Could you check a few things on this model? Use its own coordinates, in mm. A direction names the side the tool comes from. Give positions to 0.01 mm unless a question says otherwise; leave off trailing zeros. Write each loop counter-clockwise with the first axis right and the second up, starting at its lowest first coordinate (ties: lowest second). Pieces come first, ordered by that corner, then holes. Notation, with made-up numbers: M 23,53 L 33,53 A32 ccw 33,88 Z; hole C 79.5,-13.75 d6. An arc over 180 degrees is marked long. One line per item, written item: value.
```python
from build123d import *
from OCP.BRepFilletAPI import BRepFilletAPI_MakeChamfer

# Parameters (mm, degrees)
BOSS_EXTRUDE1_DEPTH      = 7
SKETCH2_R                = 1.5
CUT_EXTRUDE1_DEPTH       = 43.613787576
SKETCH3_R                = 1.5
CUT_EXTRUDE2_DEPTH       = 5
CHAMFER1_SIZE            = 0.5
CHAMFER1_SIZE2           = 0.595876796
BOSS_EXTRUDE2_DEPTH      = 2.5
BOSS_EXTRUDE2_DEPTH_BACK = 2.5
FILLET1_R                = 5
FILLET2_START            = -2.004201681
FILLET2_DEPTH            = 7.008403362
FILLET2_START_2          = 15
FILLET2_2_DEPTH          = 3


with BuildPart() as part:
    # Sketch1 → Boss-Extrude1 (new body)
    with BuildSketch(Plane(origin=(0, 0, 0), x_dir=(1, 0, 0), z_dir=(0, 1, 0))):
        with BuildLine():
            Line((15, 2.004201681), (-15, 2.004201681))
            Line((-15, 2.004201681), (-15, -2.004201681))
            Line((-15, -2.004201681), (-4, -2.004201681))
            Line((-4, -2.004201681), (-4, -37.495798319))
            Line((-4, -37.495798319), (-1, -37.495798319))
            Line((-1, -37.495798319), (-1, -30.895798319))
            ThreePointArc((-1, -30.895798319), (0, -25.895798319), (1, -30.895798319))
            Line((1, -30.895798319), (1, -37.495798319))
            Line((1, -37.495798319), (4, -37.495798319))
            Line((4, -37.495798319), (4, -2.004201681))
            Line((4, -2.004201681), (15, -2.004201681))
            Line((15, -2.004201681), (15, 2.004201681))
        make_face()
    extrude(amount=BOSS_EXTRUDE1_DEPTH)

    # Sketch2 → Cut-Extrude1 (cut, through all)
    with BuildSketch(Plane(origin=(4, 0, 0), x_dir=(0, 0, -1), z_dir=(1, 0, 0))):
        with Locations((-33.395798319, 3.5)):
            Circle(SKETCH2_R)
    extrude(amount=-CUT_EXTRUDE1_DEPTH, mode=Mode.SUBTRACT)

    # Sketch3 → Cut-Extrude2 (cut)
    with BuildSketch(Plane.XY.offset(2.004201681)):
        with Locations((9, 3.5)):
            Circle(SKETCH3_R)
        with Locations(Location((-9, 3.5, 0), (0, 0, 180))):
            Circle(SKETCH3_R)
    extrude(amount=-CUT_EXTRUDE2_DEPTH, mode=Mode.SUBTRACT)

    # Chamfer1: one chamfer whose edges measure the first distance from different faces: ONE call of the kernel's chamfer builder (chamfer() names one face for all edges)
    chamfer1_edges_1 = [part.edges().sort_by_distance(p)[0] for p in [
        (-1, 0, 34.195798319),
    ]]
    chamfer1_side_1 = [part.faces().sort_by_distance(p)[0] for p in [
        (-1, 3.5, 37.399590212),
    ]]
    chamfer1_edges_2 = [part.edges().sort_by_distance(p)[0] for p in [
        (-2.5, 0, 37.495798319),
    ]]
    chamfer1_side_2 = [part.faces().sort_by_distance(p)[0] for p in [
        (-2.5, 3.5, 37.495798319),
    ]]
    chamfer1_edges_3 = [part.edges().sort_by_distance(p)[0] for p in [
        (-4, 0, 19.75),
    ]]
    chamfer1_side_3 = [part.faces().sort_by_distance(p)[0] for p in [
        (-4, 3.5, 19.350383526),
    ]]
    chamfer1_edges_4 = [part.edges().sort_by_distance(p)[0] for p in [
        (-9.5, 0, 2.004201681),
    ]]
    chamfer1_side_4 = [part.faces().sort_by_distance(p)[0] for p in [
        (-14.869615952, 3.5, 2.004201681),
    ]]
    chamfer1_edges_5 = [part.edges().sort_by_distance(p)[0] for p in [
        (-15, 0, 0),
    ]]
    chamfer1_side_5 = [part.faces().sort_by_distance(p)[0] for p in [
        (-15, 3.5, 0),
    ]]
    chamfer1_edges_6 = [part.edges().sort_by_distance(p)[0] for p in [
        (0, 0, -2.004201681),
    ]]
    chamfer1_side_6 = [part.faces().sort_by_distance(p)[0] for p in [
        (0, 3.5, -2.004201681),
    ]]
    chamfer1_edges_7 = [part.edges().sort_by_distance(p)[0] for p in [
        (15, 0, 0),
    ]]
    chamfer1_side_7 = [part.faces().sort_by_distance(p)[0] for p in [
        (15, 3.5, 0),
    ]]
    chamfer1_edges_8 = [part.edges().sort_by_distance(p)[0] for p in [
        (9.5, 0, 2.004201681),
    ]]
    chamfer1_side_8 = [part.faces().sort_by_distance(p)[0] for p in [
        (4.130384048, 3.5, 2.004201681),
    ]]
    chamfer1_edges_9 = [part.edges().sort_by_distance(p)[0] for p in [
        (4, 0, 19.75),
    ]]
    chamfer1_side_9 = [part.faces().sort_by_distance(p)[0] for p in [
        (4, 3.5, 19.350383526),
    ]]
    chamfer1_edges_10 = [part.edges().sort_by_distance(p)[0] for p in [
        (2.5, 0, 37.495798319),
    ]]
    chamfer1_side_10 = [part.faces().sort_by_distance(p)[0] for p in [
        (2.5, 3.5, 37.495798319),
    ]]
    chamfer1_edges_11 = [part.edges().sort_by_distance(p)[0] for p in [
        (1, 0, 34.195798319),
    ]]
    chamfer1_side_11 = [part.faces().sort_by_distance(p)[0] for p in [
        (1, 3.5, 30.992006427),
    ]]
    chamfer1_edges_12 = [part.edges().sort_by_distance(p)[0] for p in [
        (0, 0, 25.895798319),
    ]]
    chamfer1_side_12 = [part.faces().sort_by_distance(p)[0] for p in [
        (0, 3.5, 25.895798319),
    ]]
    chamfer1 = BRepFilletAPI_MakeChamfer(part.part.solid().wrapped)
    for e in chamfer1_edges_1:
        chamfer1.Add(CHAMFER1_SIZE, CHAMFER1_SIZE2, e.wrapped, chamfer1_side_1[0].wrapped)  # the first distance lies on this face
    for e in chamfer1_edges_2:
        chamfer1.Add(CHAMFER1_SIZE, CHAMFER1_SIZE2, e.wrapped, chamfer1_side_2[0].wrapped)  # the first distance lies on this face
    for e in chamfer1_edges_3:
        chamfer1.Add(CHAMFER1_SIZE, CHAMFER1_SIZE2, e.wrapped, chamfer1_side_3[0].wrapped)  # the first distance lies on this face
    for e in chamfer1_edges_4:
        chamfer1.Add(CHAMFER1_SIZE, CHAMFER1_SIZE2, e.wrapped, chamfer1_side_4[0].wrapped)  # the first distance lies on this face
    for e in chamfer1_edges_5:
        chamfer1.Add(CHAMFER1_SIZE, CHAMFER1_SIZE2, e.wrapped, chamfer1_side_5[0].wrapped)  # the first distance lies on this face
    for e in chamfer1_edges_6:
        chamfer1.Add(CHAMFER1_SIZE, CHAMFER1_SIZE2, e.wrapped, chamfer1_side_6[0].wrapped)  # the first distance lies on this face
    for e in chamfer1_edges_7:
        chamfer1.Add(CHAMFER1_SIZE, CHAMFER1_SIZE2, e.wrapped, chamfer1_side_7[0].wrapped)  # the first distance lies on this face
    for e in chamfer1_edges_8:
        chamfer1.Add(CHAMFER1_SIZE, CHAMFER1_SIZE2, e.wrapped, chamfer1_side_8[0].wrapped)  # the first distance lies on this face
    for e in chamfer1_edges_9:
        chamfer1.Add(CHAMFER1_SIZE, CHAMFER1_SIZE2, e.wrapped, chamfer1_side_9[0].wrapped)  # the first distance lies on this face
    for e in chamfer1_edges_10:
        chamfer1.Add(CHAMFER1_SIZE, CHAMFER1_SIZE2, e.wrapped, chamfer1_side_10[0].wrapped)  # the first distance lies on this face
    for e in chamfer1_edges_11:
        chamfer1.Add(CHAMFER1_SIZE, CHAMFER1_SIZE2, e.wrapped, chamfer1_side_11[0].wrapped)  # the first distance lies on this face
    for e in chamfer1_edges_12:
        chamfer1.Add(CHAMFER1_SIZE, CHAMFER1_SIZE2, e.wrapped, chamfer1_side_12[0].wrapped)  # the first distance lies on this face
    add(Compound.cast(chamfer1.Shape()), mode=Mode.REPLACE)

    # Sketch4 → Boss-Extrude2 (add, two sides: drawn at the far end of the back side and taken through both)
    with BuildSketch(Plane(origin=(0, 3.5, 0), x_dir=(1, 0, 0), z_dir=(0, 1, 0)).offset(-BOSS_EXTRUDE2_DEPTH_BACK)):
        with BuildLine():
            Line((20, -23.382400921), (20, 2.004201681))
            Line((20, 2.004201681), (15, 2.004201681))
            Line((15, 2.004201681), (15, -28.382400921))
            ThreePointArc((15, -28.382400921), (16.464466094, -24.846867015), (20, -23.382400921))
        make_face()
        with BuildLine():
            Line((25, 2.004201681), (20, 2.004201681))
            Line((20, 2.004201681), (20, -23.382400921))
            ThreePointArc((20, -23.382400921), (23.535533906, -24.846867015), (25, -28.382400921))
            Line((25, -28.382400921), (25, 2.004201681))
        make_face()
        with BuildLine():
            ThreePointArc((25, -28.382400921), (23.535533906, -24.846867015), (20, -23.382400921))
            Line((20, -23.382400921), (20, -25.882400921))
            ThreePointArc((20, -25.882400921), (21.767766953, -26.614633968), (22.5, -28.382400921))
            ThreePointArc((22.5, -28.382400921), (21.767766953, -30.150167874), (20, -30.882400921))
            Line((20, -30.882400921), (20, -33.382400921))
            ThreePointArc((20, -33.382400921), (23.535533906, -31.917934827), (25, -28.382400921))
        make_face()
        with BuildLine():
            Line((20, -25.882400921), (20, -23.382400921))
            ThreePointArc((20, -23.382400921), (16.464466094, -24.846867015), (15, -28.382400921))
            ThreePointArc((15, -28.382400921), (16.464466094, -31.917934827), (20, -33.382400921))
            Line((20, -33.382400921), (20, -30.882400921))
            ThreePointArc((20, -30.882400921), (17.5, -28.382400921), (20, -25.882400921))
        make_face()
    extrude(amount=BOSS_EXTRUDE2_DEPTH + BOSS_EXTRUDE2_DEPTH_BACK)

    # Fillet1
    # the kernel refuses this fillet: 5 mm, written as the material it adds along each edge
    with BuildSketch(Plane(origin=(15, 6, -2.004201681), x_dir=(0, 1, 0), z_dir=(0, 0, 1))) as fillet1_piece_1:
        with BuildLine():
            CenterArc((5, -3), FILLET1_R, 143.130102354, 36.869897646)
            Line((0, -3), (0, 0))
            Line((0, 0), (1, 0))
        make_face()
    extrude(amount=4.008403361)
    # the kernel refuses this fillet: 5 mm, written as the material it takes off along each edge
    with BuildSketch(Plane(origin=(15, 0.5, 5.998839323), x_dir=(-0.7660444431189789, -0.6427876096865383, 0), z_dir=(0, 0, -1))) as fillet1_2_piece_1:
        with BuildLine():
            CenterArc((1.597855057, 5), FILLET1_R, 247.427648729, 22.572351271)
            Line((-0.321393805, 0.383022222), (0, 0))
            Line((0, 0), (1.597855057, 0))
        make_face()
    extrude(amount=11.997678646, mode=Mode.SUBTRACT)

    # Fillet2: read off the stored shape, not the designer's step
    # Fillet2 outline → Fillet2 (add)
    with BuildSketch(Plane.XY.offset(FILLET2_START)):
        with BuildLine():
            ThreePointArc((18, 6), (16.41886117, 6.25658351), (15, 7))
            Line((15, 7), (15, 6))
            Line((15, 6), (18, 6))
        make_face()
    extrude(amount=FILLET2_DEPTH)

    # Fillet2 2 outline → Fillet2 2 (cut)
    with BuildSketch(Plane.YZ.offset(FILLET2_START_2)):
        with BuildLine():
            Line((9, 5.004201681), (6, 5.004201681))
            ThreePointArc((6, 5.004201681), (6.25658351, 3.423062851), (7, 2.004201681))
            Line((7, 2.004201681), (7.75315126, 1))
            Line((7.75315126, 1), (9, 1))
            Line((9, 1), (9, 5.004201681))
        make_face()
    extrude(amount=FILLET2_2_DEPTH, mode=Mode.SUBTRACT)


solid = part.part
```
1) We'd pull the mould along Y, two halves only. Please class faces 1 (the face through (7.5, 3.57, 0.03)), 2 (the face through (0, 0, 12)), 3 (the face through (25, 3, 13)), 4 (the face through (0, 7, 13)): pulls with the +Y half, pulls with the -Y half, needs draft (parallel to the pull), parting line crosses it, or undercut.
Outcome:
face 1: undercut
face 2: pulls with the -Y half
face 3: needs draft
face 4: pulls with the +Y half
2) If we section it at C-C, the plane x = -9: Write out the boundary of the cut face in (y, z).
Outcome:
outline: M 0,-1.41 L 0.5,-2 L 2,-2 L 2,2 L 0.5,2 L 0,1.41 Z; M 5,-2 L 7,-2 L 7,2 L 5,2 Z
3) If we section it at D-D, the plane x = 6: Write out the boundary of the cut face in (y, z).
Outcome:
outline: M 0,-1.41 L 0.5,-2 L 7,-2 L 7,2 L 0.5,2 L 0,1.41 Z
4) I'm going to push flat-ended pins straight in: pin 1 (2 mm diameter, centred on y = 2, z = 35.5, fed in from -X); pin 2 (3.5 mm diameter, centred on y = 3.5, z = 33.4, fed in from +X); pin 3 (5 mm diameter, centred on x = 22, z = 19, fed in from +Y); pin 4 (2.5 mm diameter, centred on x = 9, y = 3.5, fed in from +Z). Where does each tip first touch, or does it pass through?
Outcome:
pin 1: stops at x = -4
pin 2: stops at x = 23.78
pin 3: stops at y = 6
pin 4: passes through
5) If we section it at A-A, the plane y = 3.5: Give the number of separate pieces and of enclosed holes in the cut face, then the cut area to 3 significant figures.
Outcome:
separate pieces: 5
enclosed holes: 1
area: 651 mm^2
6) Please list where these lines run through material, in increasing order: L1, parallel to X at y = 2.5, z = 8; L2, parallel to Y at x = -9, z = -0.7; L3, parallel to X at y = 1.5, z = 34. Write a range as from..to.
Outcome:
L1: x = -4..4, 15..25
L2: y = 0..2, 5..7
L3: x = -4..-1, 1..4
7) On a 3-axis mill with a long thin cutter (end or side, diameter ignored), from which of +Z, -Z, +X, -X, +Y, -Y can I reach the whole of each face in a straight line? I mean faces 5 (the face through (20, 6, 15)), 6 (the face through (-11, 4, 2.004)), 7 (the face through (15, 3, 15)), 8 (the face through (2.521, 3.951, 31.965)). Say none if no direction works.
Outcome:
face 5: +Z, +X, +Y
face 6: +Z, -X, +Y, -Y
face 7: +Z, +Y, -Y
face 8: -X
8) If we section it at B-B, the plane z = 15: Write out the boundary of the cut face in (x, y), then the cut area to 3 significant figures.
Outcome:
outline: M -4,0.5 L -3.4,0 L 3.4,0 L 4,0.5 L 4,7 L -4,7 Z; M 15,1 L 25,1 L 25,6 L 15,6 Z
area: 106 mm^2
